Input: part model. Units: mm. Frame: model coordinates. A direction names the side the tool comes from. Round coordinates to 2 decimals unless told otherwise and drop trailing zeros. Use a Markdown table: item, result.
from build123d import *

# Parameters (mm, degrees)
ESTRUSIONE_ESTRUSIONE1_DEPTH                         = 3
ESTRUSIONE_ESTRUSIONE1_DEPTH_BACK                    = 12
TAGLIO_ESTRUSIONE1_DEPTH                             = 3
FORO_LAMATO_PER_VITE_M6_A_TESTA_CILINDRI_D           = 6.4
FORO_LAMATO_PER_VITE_M6_A_TESTA_CILINDRI_CBORE_D     = 11
FORO_LAMATO_PER_VITE_M6_A_TESTA_CILINDRI_CBORE_DEPTH = 6.4
FORO_PER_VITE_M6_1_D                                 = 6.6
TAGLIO_ESTRUSIONE2_DEPTH                             = 2
RIPETIZIONECIRCOLARE1_COUNT                          = 2


with BuildPart() as part:
    # Schizzo1 → Estrusione-Estrusione1 (new body, two sides)
    with BuildSketch(Plane.XY) as estrusione_estrusione1_sk:
        with BuildLine():
            Line((-181.4, 70), (272.3, 70))
            ThreePointArc((272.3, 70), (279.371067812, 67.071067812), (282.3, 60))
            Line((282.3, 60), (282.3, -60))
            ThreePointArc((282.3, -60), (279.371067812, -67.071067812), (272.3, -70))
            Line((272.3, -70), (-181.4, -70))
            ThreePointArc((-181.4, -70), (-188.471067812, -67.071067812), (-191.4, -60))
            Line((-191.4, -60), (-191.4, 60))
            ThreePointArc((-191.4, 60), (-188.471067812, 67.071067812), (-181.4, 70))
        make_face()
    extrude(amount=ESTRUSIONE_ESTRUSIONE1_DEPTH)
    extrude(estrusione_estrusione1_sk.sketch, amount=-ESTRUSIONE_ESTRUSIONE1_DEPTH_BACK)

    # Schizzo2 → Taglio-Estrusione1 (cut)
    with BuildSketch(Plane.XY.offset(3)):
        with BuildLine():
            Line((196.772135955, 52), (282.3, 52))
            Line((282.3, 52), (282.3, -52))
            Line((282.3, -52), (196.772135955, -52))
            ThreePointArc((196.772135955, -52), (195.955639374, -52.174258142), (195.28142397, -52.666666667))
            ThreePointArc((195.28142397, -52.666666667), (189.471572875, -52.828427125), (189.633333333, -47.01857603))
            ThreePointArc((189.633333333, -47.01857603), (190.125741858, -46.344360626), (190.3, -45.527864045))
            Line((190.3, -45.527864045), (190.3, 45.527864045))
            ThreePointArc((190.3, 45.527864045), (190.125741858, 46.344360626), (189.633333333, 47.01857603))
            ThreePointArc((189.633333333, 47.01857603), (189.471572875, 52.828427125), (195.28142397, 52.666666667))
            ThreePointArc((195.28142397, 52.666666667), (195.955639374, 52.174258142), (196.772135955, 52))
        make_face()
    taglio_estrusione1 = extrude(amount=-TAGLIO_ESTRUSIONE1_DEPTH, mode=Mode.SUBTRACT)

    # Foro lamato per Vite M6 a testa cilindri (through all)
    with Locations(Plane(origin=(0, 0, -12), x_dir=(-1, 0, 0), z_dir=(0, 0, -1))):
        with Locations((-204.3, 41.814954576), (-204.3, -25.185045424), (-274.3, -25.185045424)):
            foro_lamato_per_vite_m6_a_testa_cilindri = CounterBoreHole(FORO_LAMATO_PER_VITE_M6_A_TESTA_CILINDRI_D / 2, FORO_LAMATO_PER_VITE_M6_A_TESTA_CILINDRI_CBORE_D / 2, FORO_LAMATO_PER_VITE_M6_A_TESTA_CILINDRI_CBORE_DEPTH)

    # Foro per Vite M6-1 (through all)
    with Locations(Plane.XY.offset(3)):
        with Locations((170.45, -25), (-79.55, 25), (170.45, 25), (-79.55, -25), (120.45, -25), (120.45, 25), (70.45, 25), (70.45, -25), (20.45, 25), (20.45, -25), (-29.55, -25), (-29.55, 25)):
            Hole(FORO_PER_VITE_M6_1_D / 2)

    # Schizzo7 → Taglio-Estrusione2 (cut)
    with BuildSketch(Plane.XY.offset(3)):
        with BuildLine():
            Line((182.3, 15), (200.3, 15))
            Line((200.3, 15), (200.3, -15))
            Line((200.3, -15), (182.3, -15))
            ThreePointArc((182.3, -15), (180.885786438, -14.414213562), (180.3, -13))
            Line((180.3, -13), (180.3, 13))
            ThreePointArc((180.3, 13), (180.885786438, 14.414213562), (182.3, 15))
        make_face()
    taglio_estrusione2 = extrude(amount=-TAGLIO_ESTRUSIONE2_DEPTH, mode=Mode.SUBTRACT)

    # RipetizioneCircolare1: Taglio-Estrusione1, Foro lamato per Vite M6 a testa cilindri, Taglio-Estrusione2 ×2 about axis
    ripetizionecircolare1_axis = Axis((45.45, 0, 0), (0, 0, 1))
    add([taglio_estrusione1.rotate(ripetizionecircolare1_axis, i * 360 / RIPETIZIONECIRCOLARE1_COUNT) for i in range(1, RIPETIZIONECIRCOLARE1_COUNT)], mode=Mode.SUBTRACT)
    add([foro_lamato_per_vite_m6_a_testa_cilindri.rotate(ripetizionecircolare1_axis, i * 360 / RIPETIZIONECIRCOLARE1_COUNT) for i in range(1, RIPETIZIONECIRCOLARE1_COUNT)], mode=Mode.SUBTRACT)
    add([taglio_estrusione2.rotate(ripetizionecircolare1_axis, i * 360 / RIPETIZIONECIRCOLARE1_COUNT) for i in range(1, RIPETIZIONECIRCOLARE1_COUNT)], mode=Mode.SUBTRACT)


solid = part.part
1) Draft query along Y for faces 4 (the face through (-108.154, 23.533, -8.845)), 5 (the face through (-188.39, -67.15, -4.39)), 6 (the face through (49, 1, -12)). Return one class per face: released by +Y, released by -Y, zero draft, split by the parting line, or undercut.
Answer key:
| item | result |
|---|---|
| face 4 | undercut |
| face 5 | released by -Y |
| face 6 | zero draft |
2) Ray query, probe 1 along Y at (x, z) = (170.45, -2.75); probe 2 along Z at (x, y) = (-135, -30); probe 3 along X at (y, z) = (-37.5, 2). Return the intervals inside material, ascending.
Answer key:
| item | result |
|---|---|
| probe 1 | y = -70 to -28.3, -21.7 to 21.7, 28.3 to 70 |
| probe 2 | z = -12 to 0 |
| probe 3 | x = -99.4 to 190.3 |
3) Set-up query: faces 1 (the face through (271.34, -20.55, -8.84)), 2 (the face through (-94, 0, 1)), 3 (the face through (42, 70, -4)). Return all of +Z, -Z, +X, -X, +Y, -Y with unobstructed straight access to the full face (end or side cutting, diameter ignored); none if empty.
Answer key:
| item | result |
|---|---|
| face 1 | -Z |
| face 2 | +Z, -X |
| face 3 | +Z, -Z, +X, -X, +Y |
4) Cut plane A-A on z = -8.5. State how many separate pieces and enclosed holes the cut face has, and give its area (3 significant figures).
Answer key:
| item | result |
|---|---|
| separate pieces | 1 |
| enclosed holes | 18 |
| area | 65,300 mm^2 |
5) Contact query for flat-ended pins moving along their axis: P1, Ø9, axis at x = -113.4, y = -41.81, coming from the -Z side; P2, Ø5, axis at x = -96, y = -2, coming from the +Z side. Output: stop coordinate, or through.
Answer key:
| item | result |
|---|---|
| P1 | stops at z = -5.6 |
| P2 | stops at z = 1 |
